```python
from build123d import *

# Parameters (mm, degrees)
F1_DEPTH = 1066.8


with BuildPart() as f1:
    # F0 (on Front) → F1 (new body)
    with BuildSketch(Plane.XZ):
        with BuildLine():
            Line((0, 711.2), (0, 0))
            Line((0, 0), (1016, 0))
            Line((1016, 0), (1016, 711.2))
            Line((1016, 711.2), (812.8, 711.2))
            ThreePointArc((812.8, 711.2), (508, 406.4), (203.2, 711.2))
            Line((203.2, 711.2), (0, 711.2))
        make_face()
    extrude(amount=F1_DEPTH)


solid = f1.part
```
Verification items for the finished model (mm, model axes). Give positions to 0.01 mm unless a question says otherwise; leave off trailing zeros. Order: outer loops, then holes, each group sorted by start corner. A loop starts at its lowest first (then second) coordinate and runs counter-clockwise, first axis right, second up. Notation, with made-up numbers: M 25.25,57.25 L 70.25,57.25 A19 ccw 70.25,85.25 Z; hole C 81.25,67 d1. An arc over 180 degrees is marked long. Answer in a Markdown table with one row per item. Add a question column.
Item 1: Scan lines: probe 1 along X at (y, z) = (-189.5, 644.5); probe 2 along Z at (x, y) = (346, -620); probe 3 along Z at (x, y) = (333.5, -667.5). Record each from-to range of solid material in increasing order. Write a range as from..to.
Item 2: Mould release check, pull along X, two halves, no side actions. Record for faces 1 (the flat face through (916, -526, 711.2)), 2 (the flat face through (1016, -526, 351)), 3 (the cylindrical face through (514.702, -525.932, 406.474)): released by +X, released by -X, zero draft, split by the parting line, or undercut.
Item 3: Section check C-C, the plane x = 357. Enter the section's corners in (y, z), and give its area (3 significant figures).
Item 4: Section check B-B, the plane y = -964. Enter the section's corners in (x, z), and give its area (3 significant figures).
Item 5: Section check A-A, the plane z = 560.5. Enter the section's corners in (x, y).
Item 6: Section check D-D, the plane x = 508. Enter the section's corners in (y, z), and give its area (3 significant figures).
Item 7: Gauge pin test, flat ends, axial feed: pin 1 (4 mm diameter, centred on x = 467.5, y = -222.5, fed in from +Z); pin 2 (2 mm diameter, centred on x = 667.5, y = -921, fed in from +Z); pin 3 (6 mm diameter, centred on x = 782, y = -634.5, fed in from +Z). Record the tip position at first contact, or that the pin passes through.
Filled sheet:
| question | item | result |
|---|---|---|
| 1 | probe 1 | x = 0..210.59, 805.41..1016 |
| 1 | probe 2 | z = 0..453.02 |
| 1 | probe 3 | z = 0..461.29 |
| 2 | face 1 | zero draft |
| 2 | face 2 | released by +X |
| 2 | face 3 | undercut |
| 3 | outline | M -1066.8,0 L 0,0 L 0,446.43 L -1066.8,446.43 Z |
| 3 | area | 476,000 mm^2 |
| 4 | outline | M 0,0 L 1016,0 L 1016,711.2 L 812.8,711.2 A304.8 cw 203.2,711.2 L 0,711.2 Z |
| 4 | area | 577,000 mm^2 |
| 5 | outline | M 0,-1066.8 L 243.06,-1066.8 L 243.06,0 L 0,0 Z; M 772.94,-1066.8 L 1016,-1066.8 L 1016,0 L 772.94,0 Z |
| 6 | outline | M -1066.8,0 L 0,0 L 0,406.4 L -1066.8,406.4 Z |
| 6 | area | 434,000 mm^2 |
| 7 | pin 1 | stops at z = 409.38 |
| 7 | pin 2 | stops at z = 452.08 |
| 7 | pin 3 | stops at z = 584.02 |
